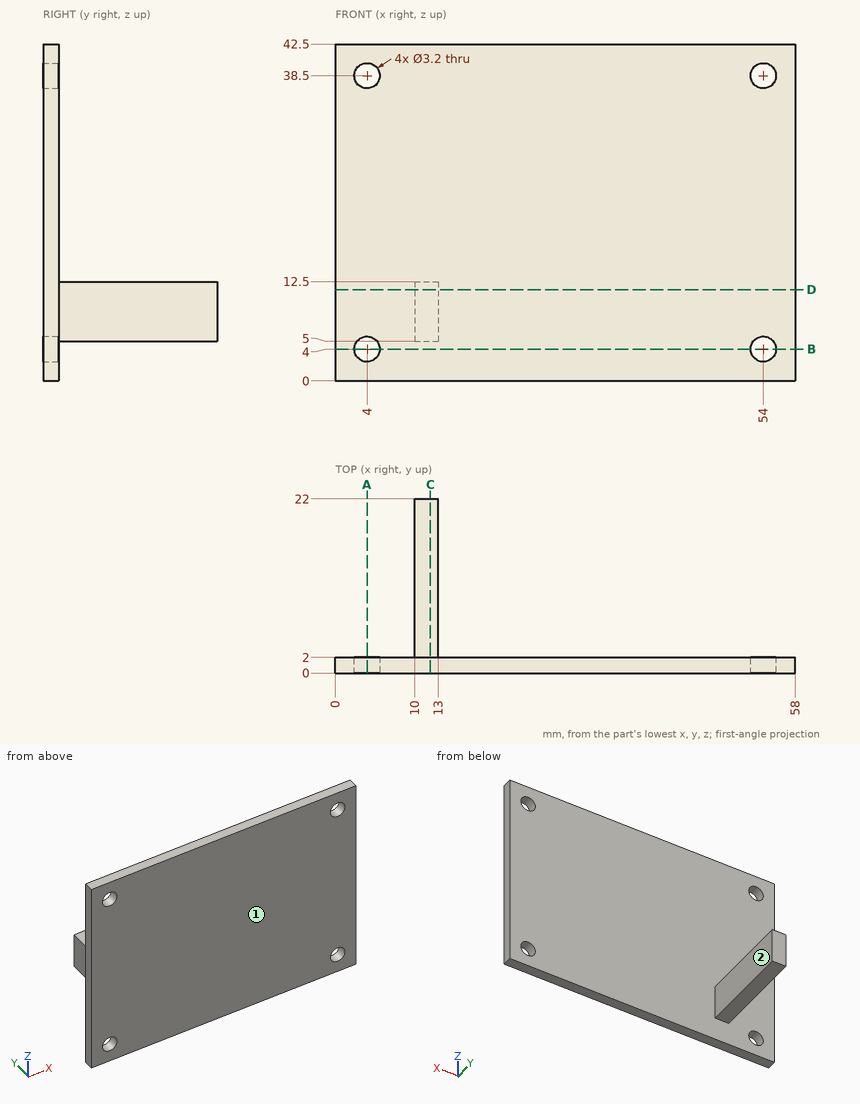
Check sheet for the drawn part. Datum: minimum x, y, z corner. Units: mm. A direction names the side the tool comes from. Give positions to 0.01 mm unless a question says otherwise; leave off trailing zeros. Order: outer loops, then holes, each group sorted by start corner. A loop starts at its lowest first (then second) coordinate and runs counter-clockwise, first axis right, second up. Notation, with made-up numbers: (7.5, 9) - (66.5, 9) arc R36 ccw to (66.5, 44) - close; hole circle Ø8 at (86, 23). An arc over 180 degrees is marked (long way). Write item = value, one per line. Start each with the question number.
1) Section check C-C (x = 12). Enter the section's corners in (y, z), then the cut area to 3 significant figures.
2) Scan lines: L1, parallel to X at y = 1.05, z = 4; L2, parallel to Z at x = 4, y = 0.9; L3, parallel to Y at x = 29.5, z = 23. Record each from-to range of solid material in increasing order.
3) Section check A-A (x = 4). Enter the section's corners in (y, z).
4) Gauge pin test, flat ends, axial feed: pin 1 Ø6 at (y, z) = (11.5, 8) entering from +X; pin 2 Ø1.5 at (x, y) = (11.5, 12) entering from -Z; pin 3 Ø4 at (x, z) = (4, 4) entering from -Y; pin 4 Ø3.5 at (x, z) = (4, 38.5) entering from +Y. Record the tip position at first contact, or that the pin passes through.
5) Section check B-B (z = 4). Enter the section's corners in (x, y), then the cut area to 3 significant figures.
6) Access from +Z, -Z, +X, -X, +Y, -Y to the whole of each face (thin tool, end or side, straight path). Record for the marked faces 1 and 2.
7) Section check D-D (z = 11.5). Enter the section's corners in (x, y), then the cut area to 3 significant figures.
Geometry check:
q1.outline = (0, 0) - (2, 0) - (2, 5) - (22, 5) - (22, 12.5) - (2, 12.5) - (2, 42.5) - (0, 42.5) - close
q1.area = 235 mm2
q2.L1 = 0 to 2.4, 5.6 to 52.4, 55.6 to 58
q2.L2 = 0 to 2.4, 5.6 to 36.9, 40.1 to 42.5
q2.L3 = 0 to 2
q3.outline = (0, 0) - (2, 0) - (2, 2.4) - (0, 2.4) - close; (0, 5.6) - (2, 5.6) - (2, 36.9) - (0, 36.9) - close; (0, 40.1) - (2, 40.1) - (2, 42.5) - (0, 42.5) - close
q4.pin_1 = 13
q4.pin_2 = 5
q4.pin_3 = 0
q4.pin_4 = 2
q5.outline = (0, 0) - (2.4, 0) - (2.4, 2) - (0, 2) - close; (5.6, 0) - (52.4, 0) - (52.4, 2) - (5.6, 2) - close; (55.6, 0) - (58, 0) - (58, 2) - (55.6, 2) - close
q5.area = 103 mm2
q6.face_1 = +Z, -Z, +X, -X, -Y
q6.face_2 = +Z, -Z, +X, +Y
q7.outline = (0, 0) - (58, 0) - (58, 2) - (13, 2) - (13, 22) - (10, 22) - (10, 2) - (0, 2) - close
q7.area = 176 mm2
